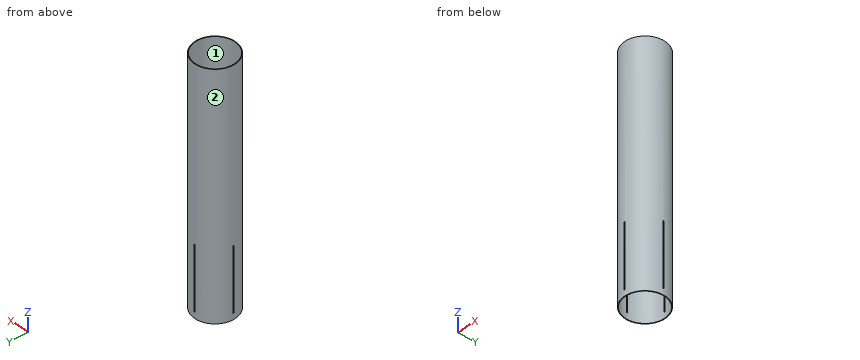
```python
from build123d import *

# Parameters (mm, degrees)
SKETCH1_R           = 65.405
SKETCH1_R_2         = 63.373
BOSS_EXTRUDE1_DEPTH = 381
SKETCH3_W           = 3.175
SKETCH3_H           = 203.2
CUT_EXTRUDE1_DEPTH  = 66.405
CIRPATTERN1_COUNT   = 4


with BuildPart() as part:
    # Sketch1 → Boss-Extrude1 (new body, symmetric)
    with BuildSketch(Plane.XY):
        Circle(SKETCH1_R)
        Circle(SKETCH1_R_2, mode=Mode.SUBTRACT)
    extrude(amount=BOSS_EXTRUDE1_DEPTH, both=True)

    # Sketch3 → Cut-Extrude1 (cut, through all)
    with BuildSketch(Plane(origin=(0, 0, 0), x_dir=(1, 0, 0), z_dir=(0, 1, 0))):
        with Locations((0, 260.35)):
            Rectangle(SKETCH3_W, SKETCH3_H)
    cut_extrude1 = extrude(amount=CUT_EXTRUDE1_DEPTH, mode=Mode.SUBTRACT)

    # CirPattern1: Cut-Extrude1 ×4 about axis
    cirpattern1_axis = Axis((0, 0, 0), (0, 0, 1))
    for i in range(1, CIRPATTERN1_COUNT):
        add(cut_extrude1.rotate(cirpattern1_axis, i * 360 / CIRPATTERN1_COUNT), mode=Mode.SUBTRACT)


solid = part.part
```
Input: part model. Units: mm. Frame: model coordinates. Face numbers are marked on the shaded views. Coordinates: 2 decimals unless noted, no trailing zeros. Loops run counter-clockwise (first coordinate to the right, second up) from the corner with the lowest first, then second, coordinate; pieces in that order, holes last. Notation, with made-up numbers: (33, 54.5) - (56, 54.5) arc R4 ccw to (56, 60.5) - close; hole circle Ø8 at (-27, -13). An arc over 180 degrees is marked (long way). Answer in a Markdown table with one row per item.
(1) Mould query, pull axis X, two halves, no side actions, for the marked faces 1 and 2. Classes: pulls with the +X half, pulls with the -X half, needs draft (parallel to the pull), parting line crosses it, or undercut.
Model answer:
| item | result |
|---|---|
| face 1 | undercut |
| face 2 | parting line crosses it |
(2) Cut plane A-A on y = 29. Output: boundary loops of the cut face in (x, z), plus the area to 3 significant figures.
Model answer:
| item | result |
|---|---|
| outline | (-58.62, -381) - (-56.35, -381) - (-56.35, 381) - (-58.62, 381) - close; (56.35, -381) - (58.62, -381) - (58.62, 381) - (56.35, 381) - close |
| area | 3,470 mm² |
(3) Material intervals for L1, parallel to Y at x = 0, z = -136 (3 decimals); L2, parallel to X at y = -29.5, z = 254, sorted ascending. Write a range as from..to.
Model answer:
| item | result |
|---|---|
| L1 | y = -65.405..-63.373, 63.373..65.405 |
| L2 | x = -58.37..-56.09, 56.09..58.37 |
(4) Pin query (flat end, axial travel): P1, Ø12, axis at y = 48.5, z = -248, coming from the -X side; P2, Ø2, axis at x = -31.5, z = -167, coming from the -Y side. Return the tip coordinate at first contact, or that it passes through.
Model answer:
| item | result |
|---|---|
| P1 | stops at x = -49.71 |
| P2 | stops at y = -57.86 |
(5) Cut plane B-B on x = -32. Output: boundary loops of the cut face in (y, z).
Model answer:
| item | result |
|---|---|
| outline | (-57.04, -381) - (-54.7, -381) - (-54.7, 381) - (-57.04, 381) - close; (54.7, -381) - (57.04, -381) - (57.04, 381) - (54.7, 381) - close |
(6) Cut plane C-C on z = -34. Output: boundary loops of the cut face in (x, y) (3 decimals), plus the area to 3 significant figures.
Model answer:
| item | result |
|---|---|
| outline | circle Ø130.81 at (0, 0); hole circle Ø126.746 at (0, 0) |
| area | 822 mm² |
